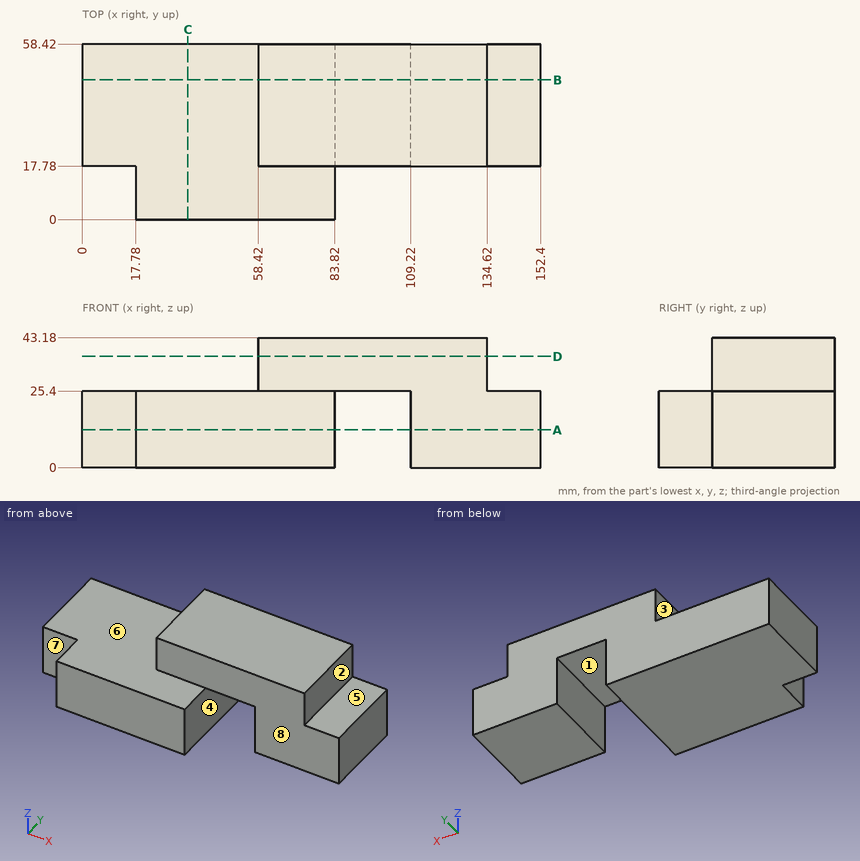
Answer from the drawing. Dimensions are ordinates in mm from the lowest x, y and z of the part. A direction names the side the tool comes from. Round coordinates to 2 decimals unless told otherwise and drop trailing zeros. Loops run counter-clockwise (first coordinate to the right, second up) from the corner with the lowest first, then second, coordinate; pieces in that order, holes last.
(1) The part is cut by section D-D, the plane z = 37. Give the vertices of the cut face in (x, y), and give its area (3 significant figures).
Computed values:
outline: (58.42, 17.78) - (134.62, 17.78) - (134.62, 58.42) - (58.42, 58.42) - close
area: 3,100 mm2
(2) Each of these flat-tipped pins is pushed along its axis until it touches: P1, Ø5.5, axis at x = 9.5, z = 7.5, coming from the -Y side; P2, Ø9, axis at y = 37.5, z = 30.5, coming from the +X side; P3, Ø17.5, axis at x = 44.5, y = 37.5, coming from the +Z side. Where does it stop, or does it pass through?
Computed values:
P1: stops at y = 17.78
P2: stops at x = 134.62
P3: stops at z = 25.4
(3) Find the intervals of material crossed by L1, parallel to X at y = 39.5, z = 5; L2, parallel to X at y = 36.5, z = 30; L3, parallel to X at y = 8, z = 2.5, in increasing order.
Computed values:
L1: x = 0 to 83.82, 109.22 to 152.4
L2: x = 58.42 to 134.62
L3: x = 17.78 to 83.82
(4) The mould has two halves that part along X. Classify the marked faces 1, 2 and 3: pulls with the +X half, pulls with the -X half, needs draft (parallel to the pull), parting line crosses it, or undercut.
Computed values:
face 1: undercut
face 2: pulls with the +X half
face 3: pulls with the -X half
(5) The part is cut by section B-B, the plane y = 46.5. Give the vertices of the cut face in (x, z), and give its area (3 significant figures).
Computed values:
outline: (0, 0) - (83.82, 0) - (83.82, 25.4) - (109.22, 25.4) - (109.22, 0) - (152.4, 0) - (152.4, 25.4) - (134.62, 25.4) - (134.62, 43.18) - (58.42, 43.18) - (58.42, 25.4) - (0, 25.4) - close
area: 4,580 mm2
(6) The part is cut by section A-A, the plane z = 12.5. Give the vertices of the cut face in (x, y).
Computed values:
outline: (0, 17.78) - (17.78, 17.78) - (17.78, 0) - (83.82, 0) - (83.82, 58.42) - (0, 58.42) - close; (109.22, 17.78) - (152.4, 17.78) - (152.4, 58.42) - (109.22, 58.42) - close
(7) For the marked faces 4, 5, 6, 7 and 8, determine the directions among +Z, -Z, +X, -X, +Y, -Y from which every point of the face is accessible in a straight line to the end or side of a thin tool.
Computed values:
face 4: -Z, +Y, -Y
face 5: +Z, +X, +Y, -Y
face 6: +Z, -X, -Y
face 7: +Z, -Z, -X, -Y
face 8: +Z, +X, -Y
(8) The part is cut by section C-C, the plane x = 35. Give the vertices of the cut face in (y, z).
Computed values:
outline: (0, 0) - (58.42, 0) - (58.42, 25.4) - (0, 25.4) - close
